```python
from build123d import *

# Parameters (mm, degrees)
SKIZZE1_R                       = 44.944071705
SKIZZE1_R_2                     = 4.923692712
AUFSATZ_LINEAR_AUSTRAGEN1_DEPTH = 5
AUFSATZ_LINEAR_AUSTRAGEN2_DEPTH = 1


with BuildPart() as part:
    # Skizze1 → Aufsatz-Linear austragen1 (new body)
    with BuildSketch(Plane.XY):
        Circle(SKIZZE1_R)
        with Locations((0, 26.9875)):
            Circle(SKIZZE1_R_2, mode=Mode.SUBTRACT)
    extrude(amount=AUFSATZ_LINEAR_AUSTRAGEN1_DEPTH)

    # Skizze2 → Aufsatz-Linear austragen2 (add)
    with BuildSketch(Plane.XY.offset(5)):
        Polygon((-1.060559395, 17.9375), (0.407051282, 17.9375), (0.407051282, 10), (-0.305288462, 10), (-0.305288462, 17.123397436), (-1.526442308, 17.123397436), align=None)
    extrude(amount=AUFSATZ_LINEAR_AUSTRAGEN2_DEPTH)


solid = part.part
```
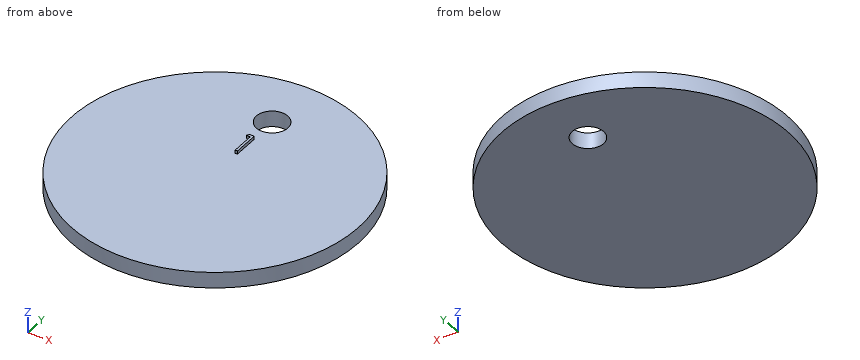
Input: part model. Units: mm. Frame: model coordinates. Coordinates: 2 decimals unless noted, no trailing zeros. Order: outer loops, then holes, each group sorted by start corner. A loop starts at its lowest first (then second) coordinate and runs counter-clockwise, first axis right, second up. Notation, with made-up numbers: (-7, 69.5) - (36, 69.5) arc R13 cw to (36, 77.5) - close; hole circle Ø10 at (80.25, 36.5). An arc over 180 degrees is marked (long way). Put each result on its own line as item: value.
1. Cut plane A-A on y = 0. Return the cut outline in (x, z).
Report:
outline: (-44.94, 0) - (44.94, 0) - (44.94, 5) - (-44.94, 5) - close
2. Cut plane B-B on z = 3.7. Return the cut outline in (x, y), then the cut area to 3 significant figures.
Report:
outline: circle Ø89.89 at (0, 0); hole circle Ø9.85 at (0, 26.99)
area: 6,270 mm2
3. Line query: line 1 along Y through (x, z) = (0, 2.35); line 2 along Z through (x, y) = (30.5, 1); line 3 along X through (y, z) = (23.5, 4.8). Output: solid intervals per line, ascending.
Report:
line 1: y = -44.94 to 22.06, 31.91 to 44.94
line 2: z = 0 to 5
line 3: x = -38.31 to -3.48, 3.48 to 38.31
4. Contact query for flat-ended pins moving along their axis: pin 1 Ø12 at (x, y) = (32.5, 1) entering from +Z; pin 2 Ø0.5 at (x, z) = (-1, 5.5) entering from -Y; pin 3 Ø0.5 at (x, z) = (0, 5.5) entering from +Y; pin 4 Ø9 at (x, y) = (0, 26.99) entering from +Z. Output: stop coordinate, or through.
Report:
pin 1: stops at z = 5
pin 2: stops at y = 17.12
pin 3: stops at y = 17.94
pin 4: passes through
5. Cut plane C-C on x = 36. Return the cut outline in (y, z).
Report:
outline: (-26.91, 0) - (26.91, 0) - (26.91, 5) - (-26.91, 5) - close
